Answer from the drawing. Dimensions are ordinates in mm from the lowest x, y and z of the part. Round coordinates to 2 decimals unless told otherwise and drop trailing zeros. Loops run counter-clockwise (first coordinate to the right, second up) from the corner with the lowest first, then second, coordinate; pieces in that order, holes last. Notation, with made-up numbers: M 78.5,-2 L 114.5,-2 A24 ccw 114.5,15 Z; hole C 58.5,29.5 d11. An arc over 180 degrees is marked long. Answer as a JSON object with one key per item and string values.
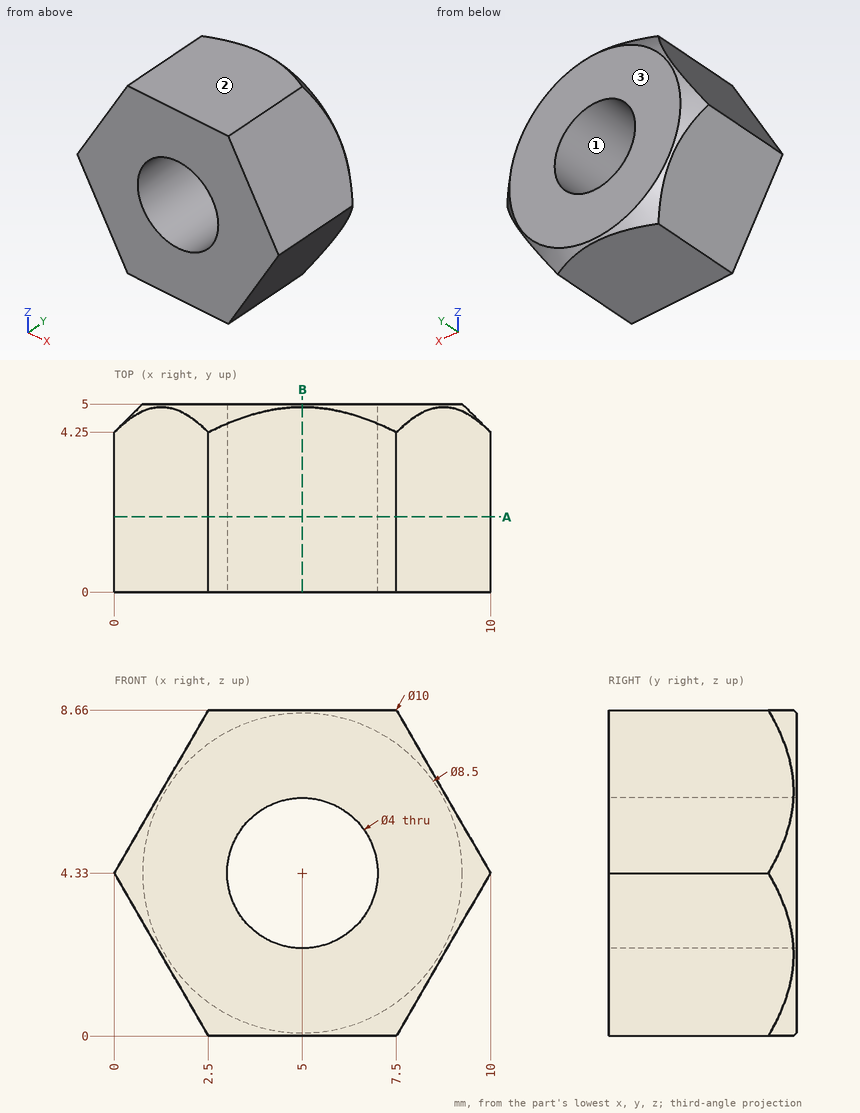
Item 1: The part is cut by section B-B (x = 5). Give the vertices of the cut face in (y, z).
Values follow:
{"outline": "M 0,0 L 4.92,0 L 5,0.08 L 5,2.33 L 0,2.33 Z; M 0,6.33 L 5,6.33 L 5,8.58 L 4.92,8.66 L 0,8.66 Z"}
Item 2: A flat-ended cylindrical pin translates along its axis: P1, Ø3, axis at x = 5, z = 4.33, coming from the -Y side. Find the tip coordinate at first contact, or state that the pin passes through.
Values follow:
{"P1": "through"}
Item 3: Determine the mould class of the marked faces 1, 2 and 3 for opening direction Z: released by +Z, released by -Z, zero draft, split by the parting line, or undercut.
Values follow:
{"face 1": "undercut", "face 2": "released by +Z", "face 3": "zero draft"}
Item 4: Straight lines are drawn through the part: line 1 (Z direction, x = 5, y = 2.55); line 2 (Z direction, x = 6.5, y = 2.15); line 3 (X direction, y = 1.5, z = 5) (1 decimal). For each, find the intervals that lie inside material, in ascending order.
Values follow:
{"line 1": "0 to 2.33, 6.33 to 8.66", "line 2": "0 to 3.01, 5.65 to 8.66", "line 3": "0.4 to 3.1, 6.9 to 9.6"}
Item 5: The part is cut by section A-A (y = 2). Give the vertices of the cut face in (x, z).
Values follow:
{"outline": "M 0,4.33 L 2.5,0 L 7.5,0 L 10,4.33 L 7.5,8.66 L 2.5,8.66 Z; hole C 5,4.33 d4"}
